Geometry: final body of the model. Coordinates: model frame, mm. Face numbers are marked on the shaded views. A direction names the side the tool comes from. Give positions to 0.01 mm unless a question says otherwise; leave off trailing zeros. Order: outer loops, then holes, each group sorted by start corner. A loop starts at its lowest first (then second) coordinate and runs counter-clockwise, first axis right, second up. Notation, with made-up numbers: (-12, -13.5) -> (14, -13.5) arc R12 ccw to (14, -8.5) -> close; hole circle Ø10 at (4.25, 14). An arc over 180 degrees is marked (long way). One line per question, with ' | ' between items.
from build123d import *

# Parameters (mm, degrees)
BOSS_EXTRUDE2_DEPTH      = 31.75
BOSS_EXTRUDE2_DEPTH_BACK = 31.75
CUT_EXTRUDE3_REACH       = 286.406
SKETCH2_R                = 82.55


with BuildPart() as part:
    # Sketch1 → Boss-Extrude2 (new, two sides: drawn at the far end of the back side and taken through both)
    with BuildSketch(Plane.XY.offset(-BOSS_EXTRUDE2_DEPTH_BACK)):
        with BuildLine():
            Line((79.549433334, -52.3875), (260.35, -52.3875))
            Line((260.35, -52.3875), (260.35, -77.7875))
            Line((260.35, -77.7875), (6.45412764, -95.031083001))
            ThreePointArc((6.45412764, -95.031083001), (-95.25, 0), (6.45412764, 95.031083001))
            Line((6.45412764, 95.031083001), (260.35, 77.7875))
            Line((260.35, 77.7875), (260.35, 52.3875))
            Line((260.35, 52.3875), (79.549433334, 52.3875))
            ThreePointArc((79.549433334, 52.3875), (95.25, 0), (79.549433334, -52.3875))
        make_face()
    extrude(amount=BOSS_EXTRUDE2_DEPTH + BOSS_EXTRUDE2_DEPTH_BACK)

    # Sketch2 → Cut-Extrude3 (cut, up to next)
    with BuildSketch(Plane.XY.offset(31.75), mode=Mode.PRIVATE) as cut_extrude3_sk1:
        Circle(SKETCH2_R)
    cut_extrude3_tool1 = extrude(cut_extrude3_sk1.sketch, amount=-CUT_EXTRUDE3_REACH, mode=Mode.PRIVATE) & part.part
    add(cut_extrude3_tool1.solids().sort_by_distance((0, 0, 31.75))[0], mode=Mode.SUBTRACT)


solid = part.part
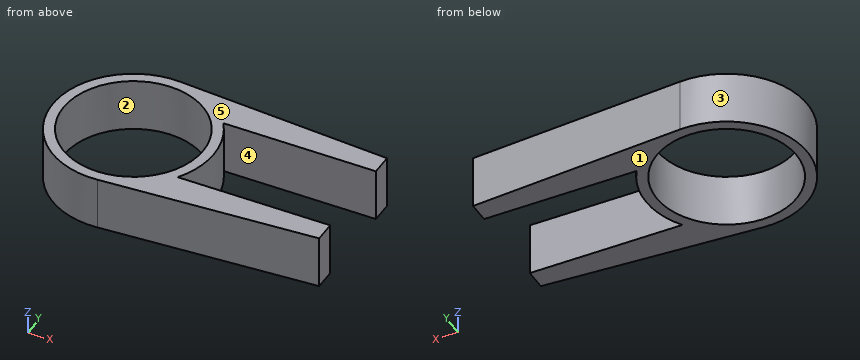
1) Section B-B on z = -5.5. Return loops of the section in (x, y), plus the area to 3 significant figures.
Check result:
outline: (6.45, -95.03) -> (260.35, -77.79) -> (260.35, -52.39) -> (79.55, -52.39) arc R95.25 ccw to (79.55, 52.39) -> (260.35, 52.39) -> (260.35, 77.79) -> (6.45, 95.03) arc R95.25 ccw (long way) to start; hole circle Ø165.1 at (0, 0) | area: 20,100 mm^2
2) Pull-direction query (Y, two-part tool) for the marked faces 1, 2 and 3; classes: +Y half, -Y half, draft (parallel to the pull), parting line (faces both ways), or undercut.
Check result:
face 1: draft | face 2: undercut | face 3: parting line
3) Material intervals for probe 1 along Y at (x, z) = (-3.5, 18.5); probe 2 along Y at (x, z) = (-26.5, -27.5), sorted ascending. Write a range as from..to.
Check result:
probe 1: y = -95.19..-82.48, 82.48..95.19 | probe 2: y = -91.49..-78.18, 78.18..91.49
4) Section A-A on y = 0. Return loops of the section in (x, z).
Check result:
outline: (-95.25, -31.75) -> (-82.55, -31.75) -> (-82.55, 31.75) -> (-95.25, 31.75) -> close; (82.55, -31.75) -> (95.25, -31.75) -> (95.25, 31.75) -> (82.55, 31.75) -> close
5) Set-up query: the marked faces 4 and 5. Return all of +Z, -Z, +X, -X, +Y, -Y with unobstructed straight access to the full face (end or side cutting, diameter ignored); none if empty.
Check result:
face 4: +Z, -Z, +X | face 5: +Z, +X, -X, +Y, -Y
6) Contact query for flat-ended pins moving along their axis: pin 1 Ø10 at (x, z) = (43, -12) entering from +Y; pin 2 Ø1 at (x, z) = (22, -4.5) entering from -Y; pin 3 Ø4 at (x, z) = (216, 13.5) entering from +Y. Output: stop coordinate, or through.
Check result:
pin 1: stops at y = 92.89 | pin 2: stops at y = -94.01 | pin 3: stops at y = 80.94
